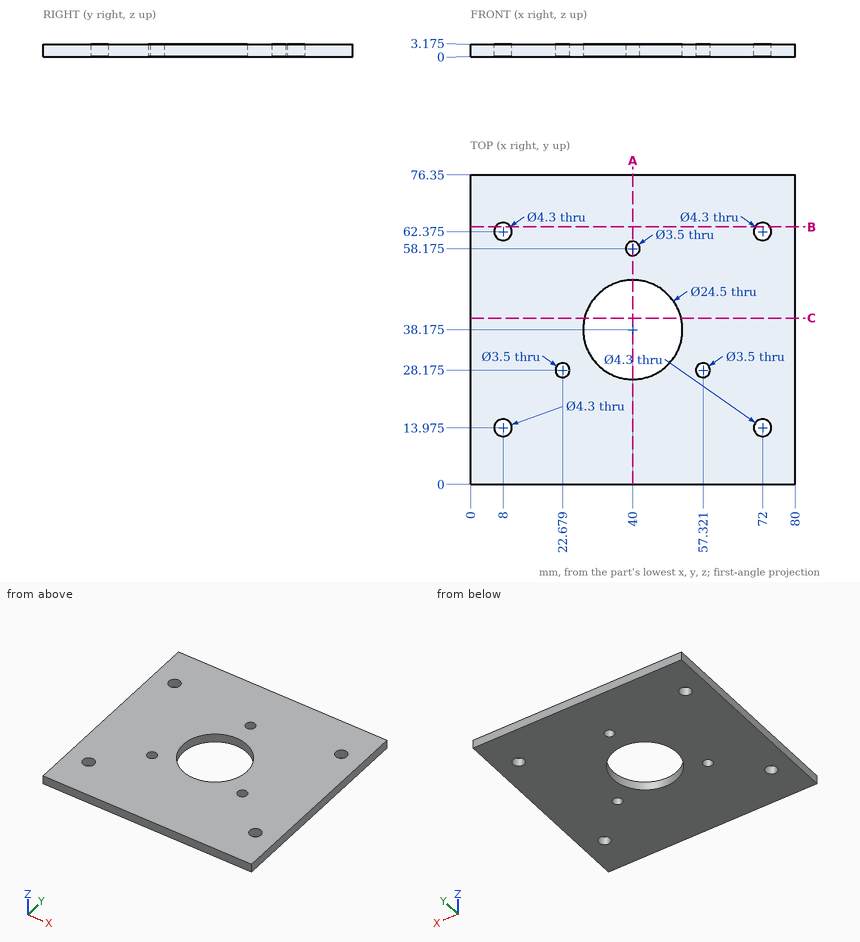
Source: three-view drawing plus pictorial views. Frame: mm from the lowest corner of the part. Round coordinates to 2 decimals unless told otherwise and drop trailing zeros. Order: outer loops, then holes, each group sorted by start corner. A loop starts at its lowest first (then second) coordinate and runs counter-clockwise, first axis right, second up. Notation, with made-up numbers: (19.5, 33.25) -> (55.5, 33.25) arc R22 cw to (55.5, 44.25) -> close; hole circle Ø6 at (-35.75, 79). An arc over 180 degrees is marked (long way). Use one line per item in the form item = value. Start each with the question number.
1. Cut plane B-B (y = 63.5). Return the cut outline in (x, z) (1 decimal).
2. Pin query (flat end, axial travel): pin 1 Ø2.5 at (x, y) = (8, 13.975) entering from -Z. Return the tip coordinate at first contact, or that it passes through.
3. Cut plane A-A (x = 40). Count the separate pieces of the cut face and the enclosed holes in it.
4. Cut plane C-C (y = 41). Return the cut outline in (x, z) (1 decimal).
5. Line query: probe 1 along X at (y, z) = (38, 3); probe 2 along X at (y, z) = (57.5, 1.1) (1 decimal); probe 3 along X at (y, z) = (61.5, 1.85) (1 decimal). Output: solid intervals per line, ascending.
Solution:
q1.outline = (0, 0) -> (6.2, 0) -> (6.2, 3.2) -> (0, 3.2) -> close; (9.8, 0) -> (70.2, 0) -> (70.2, 3.2) -> (9.8, 3.2) -> close; (73.8, 0) -> (80, 0) -> (80, 3.2) -> (73.8, 3.2) -> close
q2.pin_1 = through
q3.separate_pieces = 3
q3.enclosed_holes = 0
q4.outline = (0, 0) -> (28.1, 0) -> (28.1, 3.2) -> (0, 3.2) -> close; (51.9, 0) -> (80, 0) -> (80, 3.2) -> (51.9, 3.2) -> close
q5.probe_1 = 0 to 27.75, 52.25 to 80
q5.probe_2 = 0 to 38.4, 41.6 to 80
q5.probe_3 = 0 to 6, 10 to 70, 74 to 80
